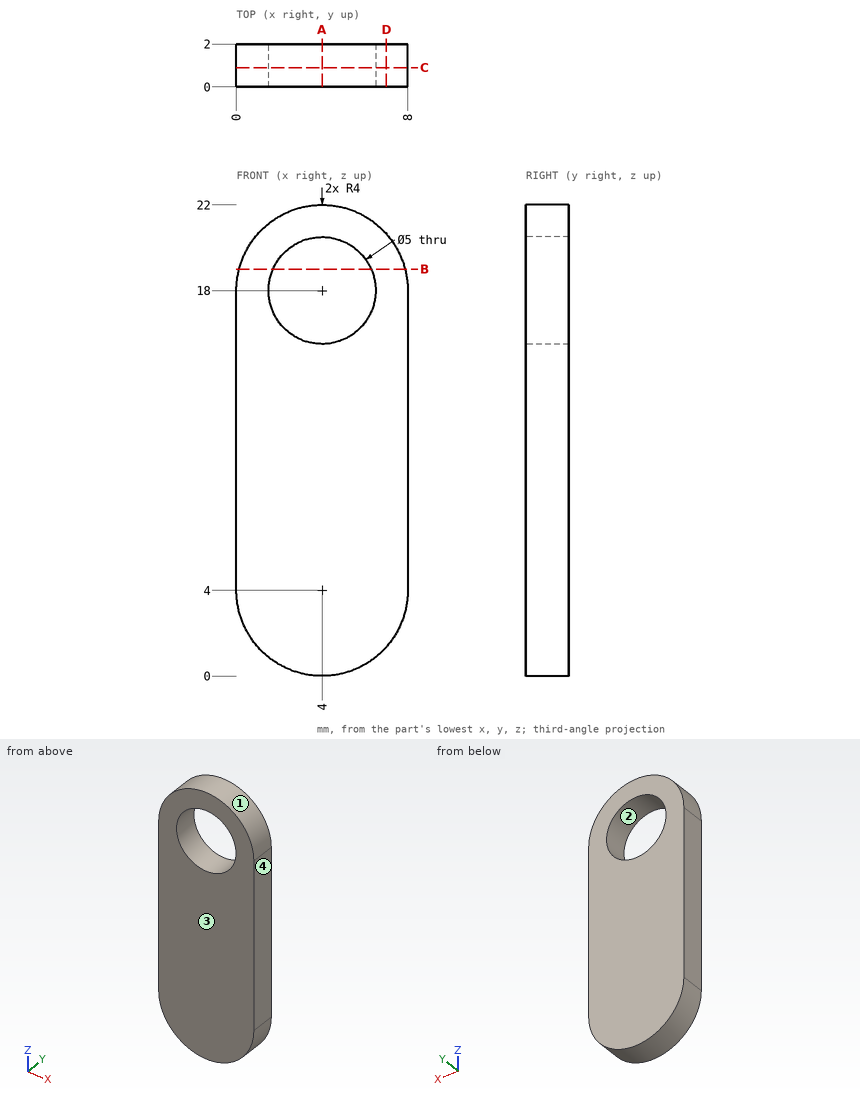
Could you check a few things on this drawing? It's one solid part, dimensions in mm from its lowest x, y, z. Give positions to 0.01 mm unless a question says otherwise; leave off trailing zeros. Write each loop counter-clockwise with the first axis right and the second up, starting at its lowest first coordinate (ties: lowest second). Pieces come first, ordered by that corner, then holes. Notation, with made-up numbers: (48, 13) -> (83, 13) arc R36 cw to (83, 52) -> close; hole circle Ø3 at (16, -30). An arc over 180 degrees is marked (long way). Answer as CSV lines item,"result". Start each with the question number.
(1) If we mould it in two halves opening along X, with no side actions, what happens to the marked faces 1, 2, 3 and 4? For each: +X half, -X half, draft (parallel to the pull), parting line (faces both ways), or undercut.
(2) If we section it at B-B, the plane z = 19: Write out the boundary of the cut face in (x, y).
(3) I'm going to push flat-ended pins straight in: pin 1 Ø2 at (x, z) = (6, 6) entering from -Y; pin 2 Ø3 at (x, z) = (4, 18) entering from +Y. Where does each tip first touch, or does it pass through?
(4) If we section it at A-A, the plane x = 4: Write out the boundary of the cut face in (y, z).
(5) If we section it at D-D, the plane x = 7: Write out the boundary of the cut face in (y, z).
(6) Please list where these lines run through material, in increasing order: line 1 (Z direction, x = 4, y = 0.9); line 2 (Z direction, x = 3.5, y = 1.85); line 3 (Z direction, x = 1.25, y = 0.85).
(7) If we section it at C-C, the plane y = 0.9: Write out the boundary of the cut face in (x, z), and give its area (3 significant figures).
Answer list:
1,face 1,"parting line"
1,face 2,"undercut"
1,face 3,"draft"
1,face 4,"+X half"
2,outline,"(0.13, 0) -> (1.71, 0) -> (1.71, 2) -> (0.13, 2) -> close; (6.29, 0) -> (7.87, 0) -> (7.87, 2) -> (6.29, 2) -> close"
3,pin 1,"y = 0"
3,pin 2,"through"
4,outline,"(0, 0) -> (2, 0) -> (2, 15.5) -> (0, 15.5) -> close; (0, 20.5) -> (2, 20.5) -> (2, 22) -> (0, 22) -> close"
5,outline,"(0, 1.35) -> (2, 1.35) -> (2, 20.65) -> (0, 20.65) -> close"
6,line 1,"0 to 15.5, 20.5 to 22"
6,line 2,"0.03 to 15.55, 20.45 to 21.97"
6,line 3,"1.1 to 20.9"
7,outline,"(0, 4) arc R4 ccw to (8, 4) -> (8, 18) arc R4 ccw to (0, 18) -> close; hole circle Ø5 at (4, 18)"
7,area,"143 mm^2"
